from build123d import *

# Parameters (mm, degrees)
SKETCH_1_W                   = 85
SKETCH_1_H                   = 98.49643328
EXTRUDE_1_DEPTH              = 2
SKETCH_1_6_W                 = 2
SKETCH_1_6_H                 = 95
EXTRUDE_2_DEPTH              = 40
SKETCH_1_7_W                 = 54
SKETCH_1_7_H                 = 2
BOSS_EXTRUDE1_DEPTH          = 15
F_10_0_START                 = -75.720313778
F_10_0_MM_DOWEL_HOLES1_DEPTH = 1.49643328
SKETCH5_W                    = 9
SKETCH5_H                    = 12
SKETCH5_W_2                  = 8
SKETCH5_H_2                  = 3.244606683
SKETCH5_W_3                  = 20
SKETCH5_H_3                  = 15
CUT_EXTRUDE1_DEPTH           = 15
SKETCH8_W                    = 25
SKETCH8_H                    = 95
SKETCH8_W_2                  = 54
SKETCH8_H_2                  = 69
CUT_EXTRUDE2_DEPTH           = 10
BOSS_EXTRUDE2_DEPTH          = 25
SKETCH11_R                   = 5.8
BOSS_EXTRUDE3_DEPTH          = 2
CAVITY1_START                = -49.696743418
CAVITY1_OUTLINE_W            = 0.5
CAVITY1_OUTLINE_H            = 3
CAVITY1_DEPTH                = 26
CAVITY1_START_2              = -38.196743418
CAVITY1_2_OUTLINE_W          = 0.5
CAVITY1_2_OUTLINE_H          = 0.5
CAVITY1_2_DEPTH              = 3
CAVITY2_START                = 0.5
CAVITY2_OUTLINE_W            = 0.5
CAVITY2_OUTLINE_H            = 3
CAVITY2_DEPTH                = 0.5


# Read off the part's stored shape, not the designer's step: Ø10.0 mm Dowel Holes1, Cavity1, Cavity2
with BuildPart() as part:
    # ｽｹｯﾁ1 → ﾎﾞｽ - 押し出し1 (new body)
    with BuildSketch(Plane(origin=(0, 0, 0), x_dir=(1, 0, 0), z_dir=(0, 1, 0))):
        with Locations((-8.696743418, 26.472097138)):
            Rectangle(SKETCH_1_W, SKETCH_1_H)
    extrude(amount=EXTRUDE_1_DEPTH)

    # ｽｹｯﾁ1<6> → ﾎﾞｽ - 押し出し2 (add)
    with BuildSketch(Plane(origin=(0, 0, 0), x_dir=(1, 0, 0), z_dir=(0, 1, 0))):
        with Locations((-50.196743418, 26.723880498)):
            Rectangle(SKETCH_1_6_W, SKETCH_1_6_H)
        Polygon((33.803256582, -20.776119502), (31.803256582, -20.776119502), (-22.196743418, -20.776119502), (-24.196743418, -20.776119502), (-49.196743418, -20.776119502), (-51.196743418, -20.776119502), (-51.196743418, -22.776119502), (33.803256582, -22.776119502), align=None)
        Polygon((-22.196743418, 74.223880498), (31.803256582, 74.223880498), (31.803256582, 75.720313778), (-51.196743418, 75.720313778), (-51.196743418, 74.223880498), (-49.196743418, 74.223880498), (-24.196743418, 74.223880498), align=None)
        Polygon((31.803256582, 50.223880498), (31.803256582, 48.223880498), (31.803256582, -20.776119502), (33.803256582, -20.776119502), (33.803256582, 75.720313778), (31.803256582, 75.720313778), (31.803256582, 74.223880498), align=None)
    extrude(amount=EXTRUDE_2_DEPTH)

    # ｽｹｯﾁ1<7> → Boss-Extrude1 (add)
    with BuildSketch(Plane(origin=(0, 0, 0), x_dir=(1, 0, 0), z_dir=(0, 1, 0))):
        with Locations((4.803256582, 49.223880498)):
            Rectangle(SKETCH_1_7_W, SKETCH_1_7_H)
        Polygon((-22.196743418, -20.776119502), (-22.196743418, 48.223880498), (-22.196743418, 50.223880498), (-22.196743418, 74.223880498), (-24.196743418, 74.223880498), (-24.196743418, -20.776119502), align=None)
    extrude(amount=BOSS_EXTRUDE1_DEPTH)

    # Ø10.0 mm Dowel Holes1 outline → Ø10.0 mm Dowel Holes1 (cut)
    with BuildSketch(Plane.XY.offset(F_10_0_START)):
        with BuildLine():
            Line((-6.31353142, 9.931926182), (-6.21353142, 9.931926182))
            ThreePointArc((-6.21353142, 9.931926182), (-0.41353142, 15.731926182), (-6.21353142, 21.531926182))
            Line((-6.21353142, 21.531926182), (-6.31353142, 21.531926182))
            ThreePointArc((-6.31353142, 21.531926182), (-12.11353142, 15.731926182), (-6.31353142, 9.931926182))
        make_face()
        with BuildLine():
            ThreePointArc((13.78646858, 9.931926182), (19.58646858, 15.731926182), (13.78646858, 21.531926182))
            Line((13.78646858, 21.531926182), (13.68646858, 21.531926182))
            ThreePointArc((13.68646858, 21.531926182), (7.88646858, 15.731926182), (13.68646858, 9.931926182))
            Line((13.68646858, 9.931926182), (13.78646858, 9.931926182))
        make_face()
    extrude(amount=F_10_0_MM_DOWEL_HOLES1_DEPTH, mode=Mode.SUBTRACT)

    # Sketch5 → Cut-Extrude1 (cut)
    with BuildSketch(Plane(origin=(0, 0, 20.776119502), x_dir=(-1, 0, 0), z_dir=(0, 0, -1))):
        with Locations((-22.303256582, 9)):
            Rectangle(SKETCH5_W, SKETCH5_H)
        with Locations((6.196743418, 4.622303342)):
            Rectangle(SKETCH5_W_2, SKETCH5_H_2)
        with Locations((36.696743418, 12.5)):
            Rectangle(SKETCH5_W_3, SKETCH5_H_3)
    extrude(amount=-CUT_EXTRUDE1_DEPTH, mode=Mode.SUBTRACT)

    # Sketch8 → Cut-Extrude2 (cut)
    with BuildSketch(Plane(origin=(0, 2, 0), x_dir=(1, 0, 0), z_dir=(0, 1, 0))):
        with Locations((-36.696743418, 26.723880498)):
            Rectangle(SKETCH8_W, SKETCH8_H)
        with Locations((4.803256582, 13.723880498)):
            Rectangle(SKETCH8_W_2, SKETCH8_H_2)
    extrude(amount=-CUT_EXTRUDE2_DEPTH, mode=Mode.SUBTRACT)



with BuildPart() as body_2:
    # Sketch9 → Boss-Extrude2 (new body)
    with BuildSketch(Plane(origin=(0, 15, 0), x_dir=(1, 0, 0), z_dir=(0, 1, 0))):
        Polygon((-22.196743418, -20.776119502), (-22.196743418, 48.223880498), (4.803256582, 48.223880498), (4.803256582, 50.223880498), (-24.196743418, 50.223880498), (-24.196743418, -20.776119502), align=None)
    extrude(amount=BOSS_EXTRUDE2_DEPTH)


with BuildPart() as part_1:
    add(part.part)

    add(body_2.part)  # Boss-Extrude3 merges body 2
    # Sketch11 → Boss-Extrude3 (add)
    with BuildSketch(Plane(origin=(0, 40, 0), x_dir=(1, 0, 0), z_dir=(0, 1, 0))):
        Polygon((31.803256582, 48.223880498), (-22.196743418, 48.223880498), (-22.196743418, 9.365118158), (-22.196743418, -20.776119502), (31.803256582, -20.776119502), align=None)
        with Locations(Location((-8.696743418, 9.365118158, 0), (0, 0, 270))):
            Circle(SKETCH11_R, mode=Mode.SUBTRACT)
    extrude(amount=-BOSS_EXTRUDE3_DEPTH)

    # Cavity1 outline → Cavity1 (cut)
    with BuildSketch(Plane.YZ.offset(CAVITY1_START)):
        with Locations((0.75, -7.451121589)):
            Rectangle(CAVITY1_OUTLINE_W, CAVITY1_OUTLINE_H)
        with Locations((0.75, -32.451121589)):
            Rectangle(CAVITY1_OUTLINE_W, CAVITY1_OUTLINE_H)
        with Locations((0.75, -57.451121589)):
            Rectangle(CAVITY1_OUTLINE_W, CAVITY1_OUTLINE_H)
    extrude(amount=CAVITY1_DEPTH, mode=Mode.SUBTRACT)

    # Cavity1 2 outline → Cavity1 2 (cut)
    with BuildSketch(Plane.YZ.offset(CAVITY1_START_2)):
        with Locations((0.75, 21.026119502)):
            Rectangle(CAVITY1_2_OUTLINE_W, CAVITY1_2_OUTLINE_H)
    extrude(amount=CAVITY1_2_DEPTH, mode=Mode.SUBTRACT)

    # Cavity2 outline → Cavity2 (cut)
    with BuildSketch(Plane(origin=(0, 0, 0), x_dir=(1, 0, 0), z_dir=(0, 1, 0)).offset(CAVITY2_START)):
        Polygon((-7.196747436, 48.227352565), (-7.197904792, 48.727351226), (-10.197896755, 48.720407091), (-10.196747436, 48.223880498), (-8.696743418, 48.223880498), align=None)
        Polygon((16.802103245, 48.720407091), (16.803252564, 48.223880498), (18.303256582, 48.223880498), (19.803252564, 48.227352565), (19.802095208, 48.727351226), align=None)
        with Locations((-22.446743418, 36.723880498)):
            Rectangle(CAVITY2_OUTLINE_W, CAVITY2_OUTLINE_H)
        with Locations((32.053256582, 36.723880498)):
            Rectangle(CAVITY2_OUTLINE_W, CAVITY2_OUTLINE_H)
        with Locations((-22.446743418, 13.723880498)):
            Rectangle(CAVITY2_OUTLINE_W, CAVITY2_OUTLINE_H)
        with Locations((32.053256582, 13.723880498)):
            Rectangle(CAVITY2_OUTLINE_W, CAVITY2_OUTLINE_H)
        with Locations((-22.446743418, -9.276119502)):
            Rectangle(CAVITY2_OUTLINE_W, CAVITY2_OUTLINE_H)
        with Locations((32.053256582, -9.276119502)):
            Rectangle(CAVITY2_OUTLINE_W, CAVITY2_OUTLINE_H)
        Polygon((-8.696743418, -20.776119502), (-10.196747436, -20.776119502), (-10.197896755, -21.272646095), (-7.197904792, -21.27959023), (-7.196747436, -20.779591569), align=None)
        Polygon((19.803252564, -20.779591569), (18.303256578, -20.776119502), (16.803252564, -20.776119502), (16.802103245, -21.272646095), (19.802095208, -21.27959023), align=None)
    extrude(amount=CAVITY2_DEPTH, mode=Mode.SUBTRACT)


solid = part_1.part
Could you check a few things on this model? Use its own coordinates, in mm. A direction names the side the tool comes from. Coordinates: 2 decimals unless noted, no trailing zeros. Loops run counter-clockwise (first coordinate to the right, second up) from the corner with the lowest first, then second, coordinate; pieces in that order, holes last.
1. Imagine slicing it at A-A (z = 9). Please give me the cut outline in (x, y).
2. I need wall thicknesses on L1, parallel to X at y = 24, z = -29.5; L2, parallel to Z at x = -16, y = 37.5; L3, parallel to Z at x = -25, y = 32. Which ranges of each line are inside material? Lowest first, please.
3. Imagine slicing it at B-B (x = -41.5). Please give me the cut outline in (y, z), and give its area (3 significant figures).
4. We'd pull the mould along X, two halves only. Please class faces 1 (the face through (33.803, 20, -26)), 2 (the face through (31.803, 20, -26)), 3 (the face through (-9, 20, 22.776)), 4 (the face through (-51.197, 20, -26)): released by +X, released by -X, zero draft, split by the parting line, or undercut.
5. For P1, Ø2, axis at x = -8.5, z = -59.5, coming from the +Y side, with a flat end and sliding along its axis, tell me the tip position at first contact or that it passes through.
6. Imagine slicing it at C-C (y = 31.5). Please give me the cut outline in (x, z), and give its area (3 significant figures).
7. Imagine slicing it at D-D (z = -26). Please give me the cut outline in (x, y).
8. For faces 5 (the face through (-2, 15, -48.224)), 6 (the face through (4, 2, -62)), 7 (the face through (-0.415, 15.604, -74.983)), 8 (the face through (-49.197, 20, -26)), which set-ups out of +Z, -Z, +X, -X, +Y, -Y let a thin tool reach every point of the face, with its end or its side?
Computed values:
1. outline: (-51.2, 0) - (-49.2, 0) - (-49.2, 40) - (-51.2, 40) - close; (-24.2, 0) - (-22.2, 0) - (-22.2, 0.5) - (-22.7, 0.5) - (-22.7, 1) - (-22.2, 1) - (-22.2, 38) - (31.8, 38) - (31.8, 1) - (32.3, 1) - (32.3, 0.5) - (31.8, 0.5) - (31.8, 0) - (33.8, 0) - (33.8, 40) - (-24.2, 40) - close
2. L1: x = -51.2 to -49.2, -24.2 to -22.2, 31.8 to 33.8
2. L2: z = -75.72 to -74.22, -50.22 to -48.22, 20.78 to 22.78
2. L3: z = -75.72 to -74.22, 20.78 to 22.78
3. outline: (0, -75.72) - (40, -75.72) - (40, -74.22) - (0, -74.22) - close; (0, 20.78) - (5, 20.78) - (5, 22.78) - (0, 22.78) - close; (20, 20.78) - (40, 20.78) - (40, 22.78) - (20, 22.78) - close
3. area: 110 mm2
4. face 1: released by +X
4. face 2: undercut
4. face 3: zero draft
4. face 4: released by -X
5. P1: stops at y = 2
6. outline: (-51.2, -75.72) - (33.8, -75.72) - (33.8, 22.78) - (-51.2, 22.78) - close; hole (-49.2, -74.22) - (31.8, -74.22) - (31.8, 20.78) - (-22.2, 20.78) - (-22.2, -48.22) - (4.8, -48.22) - (4.8, -50.22) - (-24.2, -50.22) - (-24.2, 20.78) - (-49.2, 20.78) - close
6. area: 873 mm2
7. outline: (-51.2, 0) - (-49.2, 0) - (-49.2, 40) - (-51.2, 40) - close; (-24.2, 0) - (-22.2, 0) - (-22.2, 38) - (31.8, 38) - (31.8, 0) - (33.8, 0) - (33.8, 40) - (-24.2, 40) - close
8. face 5: -Y
8. face 6: +Y
8. face 7: -Z
8. face 8: +Y, -Y
